```python
from build123d import *

# Parameters (mm, degrees)
F0_R     = 2.54
F1_DEPTH = 3.175
F2_R     = 5.08
F3_R     = 2.54
F4_R     = 44.45
F5_R     = 50.8


with BuildPart() as f1:
    # F0 (on Right) → F1 (new body)
    with BuildSketch(Plane.YZ):
        Polygon((482.6, 0), (33.02, 0), (33.02, -25.4), (12.7, -25.4), (0, -25.4), (0, -152.4), (63.5, -152.4), (485.775, -38.1), (485.775, 3.175), (482.6, 3.175), align=None)
        with Locations((12.7, -127)):
            Circle(F0_R, mode=Mode.SUBTRACT)
        with BuildLine():
            ThreePointArc((15.24, -38.1), (10.903949, -39.896051), (12.7, -35.56))
            ThreePointArc((12.7, -35.56), (14.496051, -36.303949), (15.24, -38.1))
        make_face(mode=Mode.SUBTRACT)
    extrude(amount=F1_DEPTH)

    # F2
    f2_edges = [f1.edges().sort_by_distance(p)[0] for p in [
        (1.5875, 0, -152.4),
        (1.5875, 0, -25.4),
        (1.5875, 33.02, 0),
        (1.5875, 33.02, -25.4),
    ]]
    fillet(f2_edges, radius=F2_R)

    # F3
    f3_edges = [f1.edges().sort_by_distance(p)[0] for p in [
        (1.5875, 485.775, 3.175),
    ]]
    fillet(f3_edges, radius=F3_R)

    # F4
    f4_edges = [f1.edges().sort_by_distance(p)[0] for p in [
        (1.5875, 485.775, -38.1),
    ]]
    fillet(f4_edges, radius=F4_R)

    # F5
    f5_edges = [f1.edges().sort_by_distance(p)[0] for p in [
        (1.5875, 63.5, -152.4),
    ]]
    fillet(f5_edges, radius=F5_R)


solid = f1.part
```
Read the model definition and answer for the solid it produces. Units are mm, in the model's axes. Give positions to 0.01 mm unless a question says otherwise; leave off trailing zeros. Write each loop counter-clockwise with the first axis right and the second up, starting at its lowest first coordinate (ties: lowest second). Pieces come first, ordered by that corner, then holes. Notation, with made-up numbers: M -10,83 L 30,83 A25 cw 30,121 Z; hole C 51.5,-26 d2. An arc over 180 degrees is marked long. Put each result on its own line as item: value. Start each with the question number.
1. The part is cut by section C-C, the plane z = -104.5. Give the vertices of the cut face in (x, y) (3 decimals), and give its area (3 significant figures).
2. The part is cut by section B-B, the plane y = 257. Give the vertices of the cut face in (x, z) (3 decimals).
3. Consider line 1 along Z through (x, y) = (1, 12.7); line 2 along Z through (x, y) = (1.65, 22.5); line 3 along Z through (x, y) = (2.9, 148). Determine where each line is inside the solid, lowest interval first.
4. The part is cut by section A-A, the plane x = 2.55. Give the vertices of the cut face in (y, z) (3 decimals).
5. Each of these flat-tipped pins is pushed along its axis until it touches: pin 1 Ø1.6 at (x, y) = (2, 161) entering from +Z; pin 2 Ø1.6 at (x, z) = (1.5, 2) entering from -Y; pin 3 Ø1.5 at (x, z) = (2.5, -20.5) entering from -Y. Where does it stop, or does it pass through?
Final values:
1. outline: M 0,0 L 3.175,0 L 3.175,240.464 L 0,240.464 Z
1. area: 763 mm²
2. outline: M 0,-100.024 L 3.175,-100.024 L 3.175,0 L 0,0 Z
3. line 1: z = -152.4 to -129.54, -124.46 to -40.64, -35.56 to -25.4
3. line 2: z = -152.4 to -25.4
3. line 3: z = -129.53 to 0
4. outline: M 0,-147.32 A5.08 ccw 5.08,-152.4 L 56.746,-152.4 A50.8 ccw 70.019,-150.635 L 452.939,-46.988 A44.45 ccw 485.775,-4.082 L 485.775,0.635 A2.54 ccw 483.235,3.175 L 482.6,3.175 L 482.6,0 L 38.1,0 A5.08 ccw 33.02,-5.08 L 33.02,-20.32 A5.08 cw 27.94,-25.4 L 5.08,-25.4 A5.08 ccw 0,-30.48 Z; hole C 12.7,-127 d5.08; hole C 12.7,-38.1 d5.08
5. pin 1: stops at z = 0
5. pin 2: stops at y = 482.6
5. pin 3: stops at y = 32.93
